```python
from build123d import *

# Parameters (mm, degrees)
F0_W      = 73
F0_H      = 58
F1_DEPTH  = 15
F2_DEPTH  = 2
F3_W      = 5
F3_H      = 15
F4_DEPTH  = 5
F5_W      = 5
F5_H      = 15
F6_DEPTH  = 5
F7_R      = 1.25
F8_DEPTH  = 5.5
F9_DEPTH  = 5.5
F11_DEPTH = 73.001
F12_W     = 32
F12_H     = 4
F13_DEPTH = 2
F7_W      = 5
F7_H      = 5
F14_DEPTH = 3


with BuildPart() as f1:
    # F0 (on Top) → F1 (new body)
    with BuildSketch(Plane.XY):
        Rectangle(F0_W, F0_H)
        Polygon((-34.5, 18), (-34.5, 27), (34.5, 27), (34.5, 15), (34.5, -16), (34.5, -27), (-17.5, -27), (-34.5, -27), (-34.5, -18), (-34.5, 13), align=None, mode=Mode.SUBTRACT)
    extrude(amount=F1_DEPTH)

    # F0 (on Top) → F2 (join)
    with BuildSketch(Plane.XY):
        Polygon((34.5, 27), (-34.5, 27), (-34.5, 18), (-30.5, 18), (-30.5, 13), (-34.5, 13), (-34.5, -18), (-17.5, -18), (-17.5, -27), (34.5, -27), (34.5, -16), (6.203858, -16), (6.203858, 15), (18.5, 15), (18.5, 20), (21.5, 20), (21.5, 15), (34.5, 15), align=None)
    extrude(amount=F2_DEPTH)

    # F3 (on face) → F4 (join)
    with BuildSketch(Plane(origin=(0, 29, 0), x_dir=(-1, 0, 0), z_dir=(0, 1, 0))):
        with Locations((-34, 7.5)):
            Rectangle(F3_W, F3_H)
        with Locations((34, 7.5)):
            Rectangle(F3_W, F3_H)
    extrude(amount=F4_DEPTH)

    # F5 (on face) → F6 (join)
    with BuildSketch(Plane.XZ.offset(29)):
        with Locations((34, 7.5)):
            Rectangle(F5_W, F5_H)
    extrude(amount=F6_DEPTH)

    # F7 (on face) → F8 (join)
    with BuildSketch(Plane.XY.offset(15)):
        with Locations((34, -31.5)):
            Circle(F7_R)
        with Locations((-34, 31.5)):
            Circle(F7_R)
    extrude(amount=F8_DEPTH)

    # F7 (on face) → F9 (join)
    with BuildSketch(Plane.XY.offset(15)):
        with Locations((34, 31.5)):
            Circle(F7_R)
    extrude(amount=F9_DEPTH)

    # F10 (on face) → F11 (cut, through all)
    with BuildSketch(Plane.YZ.offset(36.5)):
        Polygon((-34, 0), (-29, 0), (-34, 10), align=None)
        Polygon((34, 0), (34, 10), (29, 0), align=None)
    extrude(amount=-F11_DEPTH, mode=Mode.SUBTRACT)

    # F12 (on face) → F13 (cut)
    with BuildSketch(Plane(origin=(-36.5, 0, 0), x_dir=(0, -1, 0), z_dir=(-1, 0, 0))):
        with Locations((3, 13)):
            Rectangle(F12_W, F12_H)
    extrude(amount=-F13_DEPTH, mode=Mode.SUBTRACT)

    # F7 (on face) → F14 (join)
    with BuildSketch(Plane.XY.offset(15)):
        with Locations((34, -31.5)):
            Rectangle(F7_W, F7_H)
        with Locations((34, -31.5)):
            Circle(F7_R, mode=Mode.SUBTRACT)
        with Locations((34, 31.5)):
            Rectangle(F7_W, F7_H)
        with Locations((34, 31.5)):
            Circle(F7_R, mode=Mode.SUBTRACT)
        with Locations((-34, 31.5)):
            Rectangle(F7_W, F7_H)
        with Locations((-34, 31.5)):
            Circle(F7_R, mode=Mode.SUBTRACT)
    extrude(amount=F14_DEPTH)


solid = f1.part
```
Geometry: final body of the model. Coordinates: model frame, mm. A direction names the side the tool comes from. Coordinates: 2 decimals unless noted, no trailing zeros. Order: outer loops, then holes, each group sorted by start corner. A loop starts at its lowest first (then second) coordinate and runs counter-clockwise, first axis right, second up.
Item 1: Section query D-D (x = -11.5). Output: boundary loops of the cut face in (y, z).
Answer:
outline: (-29, 0) - (29, 0) - (29, 15) - (27, 15) - (27, 2) - (-27, 2) - (-27, 15) - (-29, 15) - close
Item 2: Access query for faces 4 (the face through (-34, 29, 16)), 5 (the face through (33, -30, 18)), 6 (the face through (34.035, -31.465, 4.93)), 7 (the face through (-33, 18, 1)), 8 (the face through (34, -29, 16)). Directions: +Z, -Z, +X, -X, +Y, -Y. A direction counts if a zero-diameter tool reaches every point of the face in a straight line with its end or side. Return the directions, or none.
Answer:
face 4: +Z, +X, -X, -Y
face 5: +Z
face 6: -Z, +X, -X, -Y
face 7: +Z, -Z
face 8: +Z, +X, -X
Item 3: Section query B-B (z = 8.5). Output: boundary loops of the cut face in (x, y), then the cut area to 3 significant figures.
Answer:
outline: (-36.5, -29) - (31.5, -29) - (31.5, -33.25) - (36.5, -33.25) - (36.5, 33.25) - (31.5, 33.25) - (31.5, 29) - (-31.5, 29) - (-31.5, 33.25) - (-36.5, 33.25) - close; hole (-34.5, -27) - (34.5, -27) - (34.5, 27) - (-34.5, 27) - close
area: 572 mm2
Item 4: Section query A-A (y = 31.5). Output: boundary loops of the cut face in (x, z).
Answer:
outline: (-36.5, 5) - (-31.5, 5) - (-31.5, 18) - (-32.75, 18) - (-32.75, 20.5) - (-35.25, 20.5) - (-35.25, 18) - (-36.5, 18) - close; (31.5, 5) - (36.5, 5) - (36.5, 18) - (35.25, 18) - (35.25, 20.5) - (32.75, 20.5) - (32.75, 18) - (31.5, 18) - close
Item 5: Section query C-C (x = -22). Output: boundary loops of the cut face in (y, z).
Answer:
outline: (-29, 0) - (-27, 0) - (-27, 15) - (-29, 15) - close; (-18, 0) - (29, 0) - (29, 15) - (27, 15) - (27, 2) - (-18, 2) - close
Item 6: Contact query for flat-ended pins moving along their axis: P1, Ø2, axis at x = -28, z = 1, coming from the -Y side; P2, Ø2, axis at x = 27, z = 1.5, coming from the +Y side; P3, Ø6, axis at x = -1, y = -0.5, coming from the +Z side. Output: stop coordinate, or through.
Answer:
P1: stops at y = -29
P2: stops at y = 29
P3: stops at z = 2
Item 7: Draft query along Y for faces 1 (the face through (-34.99, 30.74, 19.23)), 2 (the face through (-36, -3, 11)), 3 (the face through (-31.5, 31, 11)). Return one class per face: released by +Y, released by -Y, zero draft, split by the parting line, or undercut.
Answer:
face 1: split by the parting line
face 2: undercut
face 3: zero draft
Item 8: Material intervals for line 1 along Y through (x, z) = (-20.5, 10); line 2 along X through (y, z) = (5, 7.75), sorted ascending.
Answer:
line 1: y = -29 to -27, 27 to 29
line 2: x = -36.5 to -34.5, 34.5 to 36.5
